CAD build for the part. Positions are in the model's coordinates, mm. Face numbers are marked on the shaded views. A direction names the side the tool comes from. Round coordinates to 2 decimals unless told otherwise and drop trailing zeros. Loops run counter-clockwise (first coordinate to the right, second up) from the corner with the lowest first, then second, coordinate; pieces in that order, holes last. Notation, with made-up numbers: M 19,31.5 L 24,31.5 A23 ccw 24,40.5 Z; hole C 24.5,60.5 d10. An arc over 180 degrees is marked long. Use one line per item in the form item = value.
from build123d import *

# Parameters (mm, degrees)
SKETCH1_R           = 30
SKETCH1_R_2         = 3
BOSS_EXTRUDE3_DEPTH = 10
SKETCH2_R           = 10
BOSS_EXTRUDE4_DEPTH = 10
SKETCH3_R           = 5
CUT_EXTRUDE1_DEPTH  = 21


with BuildPart() as part:
    # Sketch1 → Boss-Extrude3 (new body)
    with BuildSketch(Plane.XY):
        Circle(SKETCH1_R)
        with Locations((0, 21.25)):
            Circle(SKETCH1_R_2, mode=Mode.SUBTRACT)
        with Locations((21.25, 0)):
            Circle(SKETCH1_R_2, mode=Mode.SUBTRACT)
        with Locations((0, -21.25)):
            Circle(SKETCH1_R_2, mode=Mode.SUBTRACT)
        with Locations((-21.25, 0)):
            Circle(SKETCH1_R_2, mode=Mode.SUBTRACT)
    extrude(amount=BOSS_EXTRUDE3_DEPTH)

    # Sketch2 → Boss-Extrude4 (add)
    with BuildSketch(Plane(origin=(0, 0, 0), x_dir=(-1, 0, 0), z_dir=(0, 0, -1))):
        Circle(SKETCH2_R)
    extrude(amount=BOSS_EXTRUDE4_DEPTH)

    # Sketch3 → Cut-Extrude1 (cut, through all)
    with BuildSketch(Plane(origin=(0, 0, -10), x_dir=(-1, 0, 0), z_dir=(0, 0, -1))):
        Circle(SKETCH3_R)
    extrude(amount=-CUT_EXTRUDE1_DEPTH, mode=Mode.SUBTRACT)


solid = part.part
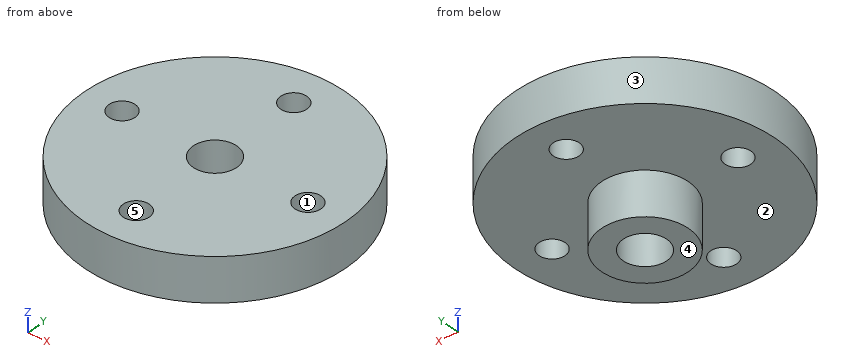
1. Pull direction Y, two halves, no side cores. Call the marked faces 3, 4 and 5: +Y half, -Y half, draft (parallel to the pull), parting line (faces both ways), or undercut.
Completed:
face_3 = parting line
face_4 = draft
face_5 = undercut
2. Cut at D-D on x = -20. Write the cut outline in (y, z).
Completed:
outline = M -22.36,0 L -2.73,0 L -2.73,10 L -22.36,10 Z; M 2.73,0 L 22.36,0 L 22.36,10 L 2.73,10 Z
3. Tool access for the marked faces 1 and 2: list every direction of +Z, -Z, +X, -X, +Y, -Y with a clear straight run to the whole face (end or side of a thin tool).
Completed:
face_1 = +Z, -Z
face_2 = -Z
4. Drop flat-ended pins along their axis: P1, Ø3, axis at y = 7.5, z = 6.5, coming from the -X side; P2, Ø3.5, axis at x = -21.25, y = 0, coming from the -Z side; P3, Ø10, axis at y = -16, z = 0, coming from the +X side; P4, Ø8, axis at y = 5, z = -7.5, coming from the -X side. Give the stop position or say it passes through.
Completed:
P1 = -29.39
P2 = through
P3 = 27.91
P4 = -9.95
5. Cut at A-A on x = 0. Write the cut outline in (y, z), and give its area (3 significant figures).
Completed:
outline = M -30,0 L -24.25,0 L -24.25,10 L -30,10 Z; M -18.25,0 L -10,0 L -10,-10 L -5,-10 L -5,10 L -18.25,10 Z; M 5,-10 L 10,-10 L 10,0 L 18.25,0 L 18.25,10 L 5,10 Z; M 24.25,0 L 30,0 L 30,10 L 24.25,10 Z
area = 480 mm2
6. Probe line 1 along Y through (x, z) = (0, 6); line 2 along Z through (x, y) = (1, -26); line 3 along Y through (x, z) = (-21.25, 6). List the from-to ranges inside material, lowest first. Write a range as from..to.
Completed:
line_1 = -30..-24.25, -18.25..-5, 5..18.25, 24.25..30
line_2 = 0..10
line_3 = -21.18..-3, 3..21.18
7. Cut at B-B on y = 23. Write the cut outline in (x, z), and give its area (3 significant figures).
Completed:
outline = M -19.26,0 L -2.44,0 L -2.44,10 L -19.26,10 Z; M 2.44,0 L 19.26,0 L 19.26,10 L 2.44,10 Z
area = 336 mm2
8. Cut at C-C on z = 2. Write the cut outline in (x, y).
Completed:
outline = C 0,0 d60; hole C -21.25,0 d6; hole C 0,0 d10; hole C 0,-21.25 d6; hole C 0,21.25 d6; hole C 21.25,0 d6
